```python
from build123d import *

# Parameters (mm, degrees)
EXTRUDE_1_DEPTH     = 2
FILLET_1_R          = 1
SKETCH_2_R          = 4
SKETCH_2_R_2        = 3
CUT_EXTRUDE_1_DEPTH = 2


with BuildPart() as part:
    # 草图1 → 凸台-拉伸1 (new body)
    with BuildSketch(Plane.XY):
        with BuildLine():
            Line((-60, 0), (0, 0))
            Line((0, 0), (0, 75.862592271))
            Line((0, 75.862592271), (0, 80))
            ThreePointArc((0, 80), (-14.574173945, 94.195139291), (-31.689992774, 83.197081668))
            Line((-31.689992774, 83.197081668), (-60, 0))
        make_face()
    extrude(amount=EXTRUDE_1_DEPTH)

    # 圆角1
    fillet_1_edges = [part.edges().sort_by_distance(p)[0] for p in [
        (0, 0, 1),
        (-60, 0, 1),
    ]]
    fillet(fillet_1_edges, radius=FILLET_1_R)

    # 草图2 → 切除-拉伸1 (cut)
    with BuildSketch(Plane.XY.offset(2)):
        with Locations((-16.214970621, 77.931296136)):
            Circle(SKETCH_2_R)
        with Locations((-10, 35)):
            Circle(SKETCH_2_R_2)
        with Locations((-10, 15)):
            Circle(SKETCH_2_R_2)
        with Locations((-45, 15)):
            Circle(SKETCH_2_R_2)
    extrude(amount=-CUT_EXTRUDE_1_DEPTH, mode=Mode.SUBTRACT)


solid = part.part
```
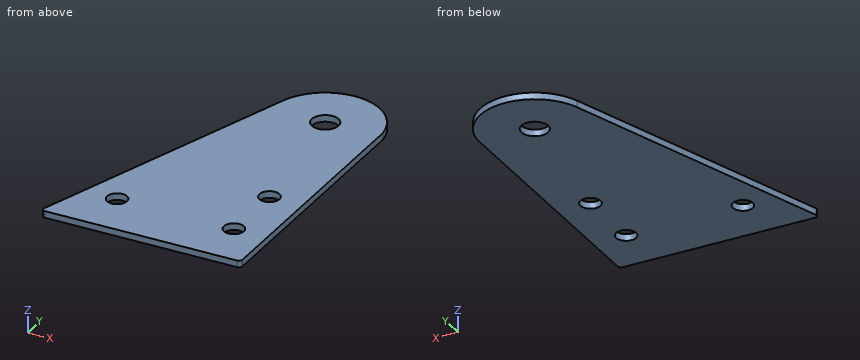
For this review, take the finished solid that the model builds, in its own axes (mm). Round coordinates to 2 decimals unless told otherwise and drop trailing zeros. Order: outer loops, then holes, each group sorted by start corner. A loop starts at its lowest first (then second) coordinate and runs counter-clockwise, first axis right, second up.
Q1. We need section D-D, the plane y = 15. Give the boundary of the cut face in (x, z).
Findings below:
outline: (-54.9, 0) - (-48, 0) - (-48, 2) - (-54.9, 2) - close; (-42, 0) - (-13, 0) - (-13, 2) - (-42, 2) - close; (-7, 0) - (0, 0) - (0, 2) - (-7, 2) - close
Q2. We need section B-B, the plane y = 33. Give the boundary of the cut face in (x, z), plus the area to 3 significant figures.
Findings below:
outline: (-48.77, 0) - (-12.24, 0) - (-12.24, 2) - (-48.77, 2) - close; (-7.76, 0) - (0, 0) - (0, 2) - (-7.76, 2) - close
area: 88.6 mm2
Q3. Wall thickness on line 1 (Y direction, x = -7.5, z = 0.95); line 2 (Y direction, x = -10, z = 1.2); line 3 (X direction, y = 12.5, z = 1.4): over which ranges is each line inside the solid? List them lowest first.
Findings below:
line 1: y = 0 to 13.34, 16.66 to 33.34, 36.66 to 91.76
line 2: y = 0 to 12, 18 to 32, 38 to 93.05
line 3: x = -55.75 to -46.66, -43.34 to -11.66, -8.34 to 0
Q4. We need section C-C, the plane z = 0.85. Give the boundary of the cut face in (x, y).
Findings below:
outline: (-59.55, 1.32) arc R1 ccw to (-58.6, 0) - (-1, 0) arc R1 ccw to (0, 1) - (0, 80) arc R16.35 ccw to (-31.69, 83.2) - close; hole circle Ø6 at (-45, 15); hole circle Ø8 at (-16.21, 77.93); hole circle Ø6 at (-10, 15); hole circle Ø6 at (-10, 35)
Q5. We need section A-A, the plane x = -45. Give the boundary of the cut face in (y, z), plus the area to 3 significant figures.
Findings below:
outline: (0, 0) - (12, 0) - (12, 2) - (0, 2) - close; (18, 0) - (44.08, 0) - (44.08, 2) - (18, 2) - close
area: 76.2 mm2
